Answer from the drawing. Dimensions are ordinates in mm from the lowest x, y and z of the part. A direction names the side the tool comes from. Coordinates: 2 decimals unless noted, no trailing zeros. Write each loop counter-clockwise with the first axis right and the second up, starting at its lowest first coordinate (ties: lowest second). Pieces come first, ordered by that corner, then holes. Notation, with made-up numbers: (27, -19) - (64, -19) arc R17 ccw to (64, -4) - close; hole circle Ø6 at (29, -0.5). An arc over 180 degrees is marked (long way). Return JSON: item names as keys, results as strings.
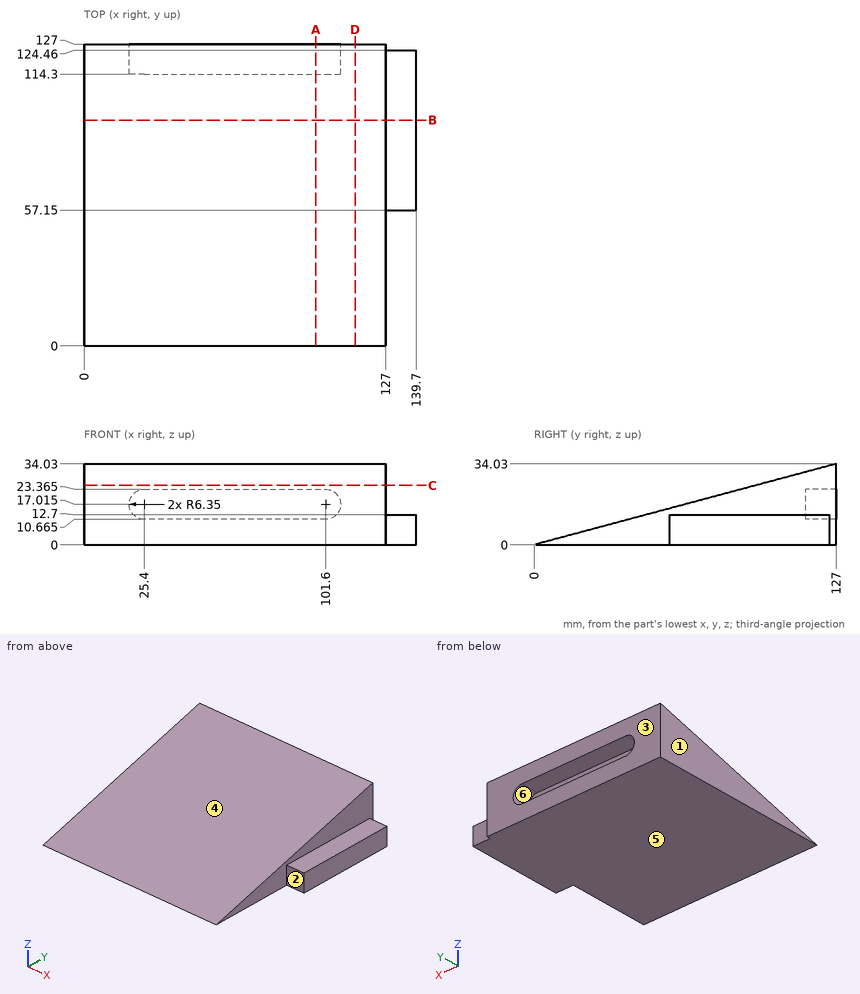
(1) A cutting plane is placed at D-D (x = 114). Determine the outline of the cut face in (y, z).
Answer:
{"outline": "(0, 0) - (127, 0) - (127, 34.03) - close"}
(2) Straight lines are drawn through the part: line 1 (X direction, y = 39.5, z = 9.5); line 2 (Z direction, x = 127.5, y = 74.5); line 3 (Z direction, x = 101, y = 113). For each, find the intervals that lie inside material, in ascending order. Write a range as from..to.
Answer:
{"line 1": "0..127", "line 2": "0..12.7", "line 3": "0..30.28"}
(3) A cutting plane is placed at C-C (z = 25). Determine the outline of the cut face in (x, y), and give its area (3 significant figures).
Answer:
{"outline": "(0, 93.3) - (127, 93.3) - (127, 127) - (0, 127) - close", "area": "4,280 mm²"}
(4) Determine the mould class of the marked faces 3, 4, 5 and 6 for opening direction Z: +Z half, -Z half, draft (parallel to the pull), parting line (faces both ways), or undercut.
Answer:
{"face 3": "draft", "face 4": "+Z half", "face 5": "-Z half", "face 6": "undercut"}
(5) A cutting plane is placed at B-B (y = 95). Determine the outline of the cut face in (x, z) (1 decimal), and give its area (3 significant figures).
Answer:
{"outline": "(0, 0) - (139.7, 0) - (139.7, 12.7) - (127, 12.7) - (127, 25.5) - (0, 25.5) - close", "area": "3,390 mm²"}
(6) Flat-ended cylindrical pins translate along their axes: P1, Ø10, axis at x = 135, z = 9, coming from the +Y side; P2, Ø14, axis at x = 136, z = 5.5, coming from the -Y side; P3, Ø4, axis at x = 42.5, z = 14, coming from the +Y side. Find the tip coordinate at first contact, or state that the pin passes through.
Answer:
{"P1": "y = 124.46", "P2": "y = 57.15", "P3": "y = 114.3"}
(7) A cutting plane is placed at A-A (x = 97.5). Determine the outline of the cut face in (y, z) (1 decimal).
Answer:
{"outline": "(0, 0) - (127, 0) - (127, 10.7) - (114.3, 10.7) - (114.3, 23.4) - (127, 23.4) - (127, 34) - close"}
(8) Which of the six approach directions +Z, -Z, +X, -X, +Y, -Y give full straight-line access (tool end or side, diameter ignored) to the marked faces 1 and 2?
Answer:
{"face 1": "+Z, -Z, -X, +Y, -Y", "face 2": "+Z, -Z, +X, -Y"}
